CAD build for the part. Positions are in the model's coordinates, mm. A direction names the side the tool comes from. Give positions to 0.01 mm unless a question says otherwise; leave off trailing zeros. Loops run counter-clockwise (first coordinate to the right, second up) from the corner with the lowest first, then second, coordinate; pieces in that order, holes last. Notation, with made-up numbers: (62.25, 30) -> (108.25, 30) arc R29 cw to (108.25, 66) -> close; hole circle Ø4 at (87.25, 20.25). An arc over 180 degrees is marked (long way). Use one line per item in the form item = value.
```python
from build123d import *
from build123d import SkipClean  # not in build123d's __all__

# Parameters (mm, degrees)
F1_DEPTH = 6
F2_DEPTH = 8
F3_DEPTH = 15
F4_DEPTH = 72
F5_DEPTH = 96
F6_DEPTH = 40
F7_R     = 4
F8_DEPTH = 25


# Not quite as in the source:
# - after a boolean that leaves OpenCascade's solid faulty, fix() repairs it


with BuildPart() as f1:
    # F0 (on Front) → F1 (new body)
    with BuildSketch(Plane.XZ):
        with BuildLine():
            Line((-21, 7.2767180102), (-21, 19.3786125664))
            ThreePointArc((-21, 19.3786125664), (-22.4015502975, 17.7398187497), (-23.6755279772, 16))
            Line((-23.6755279772, 16), (-23.6755279772, -16))
            ThreePointArc((-23.6755279772, -16), (-22.4015502975, -17.7398187497), (-21, -19.3786125664))
            Line((-21, -19.3786125664), (-21, -7.2767180102))
            ThreePointArc((-21, -7.2767180102), (-22.225, 0), (-21, 7.2767180102))
        make_face()
        with BuildLine():
            Line((-21, -7.2767180102), (-21, 7.2767180102))
            ThreePointArc((-21, 7.2767180102), (-22.225, 0), (-21, -7.2767180102))
        make_face()
        with BuildLine():
            Line((21, 7.2767180102), (21, 19.3786125664))
            ThreePointArc((21, 19.3786125664), (0, 28.575), (-21, 19.3786125664))
            Line((-21, 19.3786125664), (-21, 7.2767180102))
            ThreePointArc((-21, 7.2767180102), (0, 22.225), (21, 7.2767180102))
        make_face()
        with BuildLine():
            Line((21, -7.2767180102), (21, 7.2767180102))
            ThreePointArc((21, 7.2767180102), (0, 22.225), (-21, 7.2767180102))
            Line((-21, 7.2767180102), (-21, -7.2767180102))
            ThreePointArc((-21, -7.2767180102), (0, -22.225), (21, -7.2767180102))
        make_face()
        with BuildLine():
            ThreePointArc((10.8581766425, 9.29), (13.4046157017, 4.9518055181), (14.29, 0))
            ThreePointArc((14.29, 0), (-4.9518055181, -13.4046157017), (-10.8581766425, 9.29))
            ThreePointArc((-10.8581766425, 9.29), (0, 14.29), (10.8581766425, 9.29))
        make_face(mode=Mode.SUBTRACT)
        with BuildLine():
            ThreePointArc((-21, -19.3786125664), (0, -28.575), (21, -19.3786125664))
            Line((21, -19.3786125664), (21, -7.2767180102))
            ThreePointArc((21, -7.2767180102), (0, -22.225), (-21, -7.2767180102))
            Line((-21, -7.2767180102), (-21, -19.3786125664))
        make_face()
        with BuildLine():
            ThreePointArc((22.225, 0), (21.9166104245, 3.6895545124), (21, 7.2767180102))
            Line((21, 7.2767180102), (21, -7.2767180102))
            ThreePointArc((21, -7.2767180102), (21.9166104245, -3.6895545124), (22.225, 0))
        make_face()
        with BuildLine():
            Line((23.6755279772, -16), (23.6755279772, 16))
            ThreePointArc((23.6755279772, 16), (22.4015502975, 17.7398187497), (21, 19.3786125664))
            Line((21, 19.3786125664), (21, 7.2767180102))
            ThreePointArc((21, 7.2767180102), (21.9166104245, 3.6895545124), (22.225, 0))
            ThreePointArc((22.225, 0), (21.9166104245, -3.6895545124), (21, -7.2767180102))
            Line((21, -7.2767180102), (21, -19.3786125664))
            ThreePointArc((21, -19.3786125664), (22.4015502975, -17.7398187497), (23.6755279772, -16))
        make_face()
        with BuildLine():
            ThreePointArc((-10.8581766425, 9.29), (-4.9518055181, -13.4046157017), (14.29, 0))
            ThreePointArc((14.29, 0), (13.4046157017, 4.9518055181), (10.8581766425, 9.29))
            Line((10.8581766425, 9.29), (-10.8581766425, 9.29))
        make_face()
        with BuildLine():
            Line((-10.8581766425, 9.29), (10.8581766425, 9.29))
            ThreePointArc((10.8581766425, 9.29), (0, 14.29), (-10.8581766425, 9.29))
        make_face()
    extrude(amount=-F1_DEPTH)

    # F0 (on Front) → F2 (join)
    with BuildSketch(Plane.XZ):
        with BuildLine():
            Line((21, -7.2767180102), (21, 7.2767180102))
            ThreePointArc((21, 7.2767180102), (0, 22.225), (-21, 7.2767180102))
            Line((-21, 7.2767180102), (-21, -7.2767180102))
            ThreePointArc((-21, -7.2767180102), (0, -22.225), (21, -7.2767180102))
        make_face()
        with BuildLine():
            ThreePointArc((10.8581766425, 9.29), (13.4046157017, 4.9518055181), (14.29, 0))
            ThreePointArc((14.29, 0), (-4.9518055181, -13.4046157017), (-10.8581766425, 9.29))
            ThreePointArc((-10.8581766425, 9.29), (0, 14.29), (10.8581766425, 9.29))
        make_face(mode=Mode.SUBTRACT)
        with BuildLine():
            ThreePointArc((-10.8581766425, 9.29), (-4.9518055181, -13.4046157017), (14.29, 0))
            ThreePointArc((14.29, 0), (13.4046157017, 4.9518055181), (10.8581766425, 9.29))
            Line((10.8581766425, 9.29), (-10.8581766425, 9.29))
        make_face()
        with BuildLine():
            Line((21, 7.2767180102), (21, 19.3786125664))
            ThreePointArc((21, 19.3786125664), (0, 28.575), (-21, 19.3786125664))
            Line((-21, 19.3786125664), (-21, 7.2767180102))
            ThreePointArc((-21, 7.2767180102), (0, 22.225), (21, 7.2767180102))
        make_face()
        with BuildLine():
            ThreePointArc((-21, -19.3786125664), (0, -28.575), (21, -19.3786125664))
            Line((21, -19.3786125664), (21, -7.2767180102))
            ThreePointArc((21, -7.2767180102), (0, -22.225), (-21, -7.2767180102))
            Line((-21, -7.2767180102), (-21, -19.3786125664))
        make_face()
        with BuildLine():
            ThreePointArc((23.6755279772, -16), (27.3226905424, -8.3666723687), (28.575, 0))
            ThreePointArc((28.575, 0), (27.3226905424, 8.3666723687), (23.6755279772, 16))
            Line((23.6755279772, 16), (23.6755279772, -16))
        make_face()
        with BuildLine():
            Line((-23.6755279772, -16), (-23.6755279772, 16))
            ThreePointArc((-23.6755279772, 16), (-28.575, 0), (-23.6755279772, -16))
        make_face()
        with BuildLine():
            Line((23.6755279772, -16), (23.6755279772, 16))
            ThreePointArc((23.6755279772, 16), (22.4015502975, 17.7398187497), (21, 19.3786125664))
            Line((21, 19.3786125664), (21, 7.2767180102))
            ThreePointArc((21, 7.2767180102), (21.9166104245, 3.6895545124), (22.225, 0))
            ThreePointArc((22.225, 0), (21.9166104245, -3.6895545124), (21, -7.2767180102))
            Line((21, -7.2767180102), (21, -19.3786125664))
            ThreePointArc((21, -19.3786125664), (22.4015502975, -17.7398187497), (23.6755279772, -16))
        make_face()
        with BuildLine():
            Line((-21, 7.2767180102), (-21, 19.3786125664))
            ThreePointArc((-21, 19.3786125664), (-22.4015502975, 17.7398187497), (-23.6755279772, 16))
            Line((-23.6755279772, 16), (-23.6755279772, -16))
            ThreePointArc((-23.6755279772, -16), (-22.4015502975, -17.7398187497), (-21, -19.3786125664))
            Line((-21, -19.3786125664), (-21, -7.2767180102))
            ThreePointArc((-21, -7.2767180102), (-22.225, 0), (-21, 7.2767180102))
        make_face()
        with BuildLine():
            Line((-10.8581766425, 9.29), (10.8581766425, 9.29))
            ThreePointArc((10.8581766425, 9.29), (0, 14.29), (-10.8581766425, 9.29))
        make_face()
        with BuildLine():
            Line((-21, -7.2767180102), (-21, 7.2767180102))
            ThreePointArc((-21, 7.2767180102), (-22.225, 0), (-21, -7.2767180102))
        make_face()
        with BuildLine():
            ThreePointArc((22.225, 0), (21.9166104245, 3.6895545124), (21, 7.2767180102))
            Line((21, 7.2767180102), (21, -7.2767180102))
            ThreePointArc((21, -7.2767180102), (21.9166104245, -3.6895545124), (22.225, 0))
        make_face()
    with SkipClean():  # cleaning this boolean's faces spoils the solid; the shape is the same uncleaned
        extrude(amount=F2_DEPTH)

    # F0 (on Front) → F3 (join)
    with BuildSketch(Plane.XZ):
        with BuildLine():
            Line((21, -7.2767180102), (21, 7.2767180102))
            ThreePointArc((21, 7.2767180102), (0, 22.225), (-21, 7.2767180102))
            Line((-21, 7.2767180102), (-21, -7.2767180102))
            ThreePointArc((-21, -7.2767180102), (0, -22.225), (21, -7.2767180102))
        make_face()
        with BuildLine():
            ThreePointArc((10.8581766425, 9.29), (13.4046157017, 4.9518055181), (14.29, 0))
            ThreePointArc((14.29, 0), (-4.9518055181, -13.4046157017), (-10.8581766425, 9.29))
            ThreePointArc((-10.8581766425, 9.29), (0, 14.29), (10.8581766425, 9.29))
        make_face(mode=Mode.SUBTRACT)
        with BuildLine():
            ThreePointArc((-10.8581766425, 9.29), (-4.9518055181, -13.4046157017), (14.29, 0))
            ThreePointArc((14.29, 0), (13.4046157017, 4.9518055181), (10.8581766425, 9.29))
            Line((10.8581766425, 9.29), (-10.8581766425, 9.29))
        make_face()
        with BuildLine():
            Line((21, 7.2767180102), (21, 19.3786125664))
            ThreePointArc((21, 19.3786125664), (0, 28.575), (-21, 19.3786125664))
            Line((-21, 19.3786125664), (-21, 7.2767180102))
            ThreePointArc((-21, 7.2767180102), (0, 22.225), (21, 7.2767180102))
        make_face()
        with BuildLine():
            ThreePointArc((-21, -19.3786125664), (0, -28.575), (21, -19.3786125664))
            Line((21, -19.3786125664), (21, -7.2767180102))
            ThreePointArc((21, -7.2767180102), (0, -22.225), (-21, -7.2767180102))
            Line((-21, -7.2767180102), (-21, -19.3786125664))
        make_face()
        with BuildLine():
            Line((-10.8581766425, 9.29), (10.8581766425, 9.29))
            ThreePointArc((10.8581766425, 9.29), (0, 14.29), (-10.8581766425, 9.29))
        make_face()
    extrude(amount=F3_DEPTH)

    add(f1.part.fix(), mode=Mode.REPLACE)

    # F0 (on Front) → F4 (join)
    with BuildSketch(Plane.XZ):
        with BuildLine():
            ThreePointArc((-10.8581766425, 9.29), (-4.9518055181, -13.4046157017), (14.29, 0))
            ThreePointArc((14.29, 0), (13.4046157017, 4.9518055181), (10.8581766425, 9.29))
            Line((10.8581766425, 9.29), (-10.8581766425, 9.29))
        make_face()
        with BuildLine():
            Line((-10.8581766425, 9.29), (10.8581766425, 9.29))
            ThreePointArc((10.8581766425, 9.29), (0, 14.29), (-10.8581766425, 9.29))
        make_face()
    extrude(amount=F4_DEPTH)

    # F0 (on Front) → F5 (join)
    with BuildSketch(Plane.XZ):
        with BuildLine():
            ThreePointArc((-10.8581766425, 9.29), (-4.9518055181, -13.4046157017), (14.29, 0))
            ThreePointArc((14.29, 0), (13.4046157017, 4.9518055181), (10.8581766425, 9.29))
            Line((10.8581766425, 9.29), (-10.8581766425, 9.29))
        make_face()
    extrude(amount=F5_DEPTH)

    # F0 (on Front) → F6 (join)
    with BuildSketch(Plane.XZ):
        with BuildLine():
            Line((21, -7.2767180102), (21, 7.2767180102))
            ThreePointArc((21, 7.2767180102), (0, 22.225), (-21, 7.2767180102))
            Line((-21, 7.2767180102), (-21, -7.2767180102))
            ThreePointArc((-21, -7.2767180102), (0, -22.225), (21, -7.2767180102))
        make_face()
        with BuildLine():
            ThreePointArc((10.8581766425, 9.29), (13.4046157017, 4.9518055181), (14.29, 0))
            ThreePointArc((14.29, 0), (-4.9518055181, -13.4046157017), (-10.8581766425, 9.29))
            ThreePointArc((-10.8581766425, 9.29), (0, 14.29), (10.8581766425, 9.29))
        make_face(mode=Mode.SUBTRACT)
        with BuildLine():
            ThreePointArc((-10.8581766425, 9.29), (-4.9518055181, -13.4046157017), (14.29, 0))
            ThreePointArc((14.29, 0), (13.4046157017, 4.9518055181), (10.8581766425, 9.29))
            Line((10.8581766425, 9.29), (-10.8581766425, 9.29))
        make_face()
        with BuildLine():
            Line((-10.8581766425, 9.29), (10.8581766425, 9.29))
            ThreePointArc((10.8581766425, 9.29), (0, 14.29), (-10.8581766425, 9.29))
        make_face()
    extrude(amount=F6_DEPTH)

    # F7 (on face) → F8 (cut)
    with BuildSketch(Plane.XY.offset(9.29)):
        with Locations((0, -84)):
            Circle(F7_R)
    extrude(amount=-F8_DEPTH, mode=Mode.SUBTRACT)


solid = f1.part
```
1. Cut at B-B, the plane z = 6. Write the cut outline in (x, y), then the cut area to 3 significant figures.
Result sheet:
outline = (-27.94, -8) -> (-21, -8) -> (-21, -40) -> (-12.97, -40) -> (-12.97, -96) -> (12.97, -96) -> (12.97, -40) -> (21, -40) -> (21, -8) -> (27.94, -8) -> (27.94, 0) -> (23.68, 0) -> (23.68, 6) -> (-23.68, 6) -> (-23.68, 0) -> (-27.94, 0) -> close; hole circle Ø8 at (0, -84)
area = 3,480 mm^2
2. Mould opens along Y. For faces 6 (the cylindrical face through (0.38, -27.32, 22.22)), 7 (the cylindrical face through (-0.867, -87.905, -2.335)), 8 (the flat face through (0, 6, 0)), 9 (the flat face through (0, -40, -15)) say: pulls with the +Y half, pulls with the -Y half, needs draft (parallel to the pull), parting line crosses it, or undercut.
Result sheet:
face_6 = needs draft
face_7 = undercut
face_8 = pulls with the +Y half
face_9 = pulls with the -Y half
3. Cut at A-A, the plane x = 0. Write the cut outline in (y, z) (3 decimals), then the cut area to 3 significant figures.
Result sheet:
outline = (-96, -14.29) -> (-88, -14.29) -> (-88, 9.29) -> (-96, 9.29) -> close; (-80, -14.29) -> (-40, -14.29) -> (-40, -22.225) -> (-15, -22.225) -> (-15, -28.575) -> (6, -28.575) -> (6, 28.575) -> (-15, 28.575) -> (-15, 22.225) -> (-40, 22.225) -> (-40, 14.29) -> (-72, 14.29) -> (-72, 9.29) -> (-80, 9.29) -> close
area = 3,600 mm^2
4. Cut at C-C, the plane y = -84. Write the cut outline in (x, z), then the cut area to 3 significant figures.
Result sheet:
outline = (-10.86, 9.29) arc R14.29 ccw to (-4, -13.72) -> (-4, 9.29) -> close; (4, -13.72) arc R14.29 ccw to (10.86, 9.29) -> (4, 9.29) -> close
area = 379 mm^2
5. Cut at D-D, the plane y = -47. Write the cut outline in (x, z), then the cut area to 3 significant figures.
Result sheet:
outline = circle Ø28.58 at (0, 0)
area = 642 mm^2
6. Tool access for faces 1 (the flat face through (26, 0, 0)), 2 (the flat face through (-26, 0, 0)), 3 (the flat face through (-24, -8, 0)), 4 (the flat face through (0, -72, 11)), 5 (the flat face through (24, -8, 0)): list every direction of +Z, -Z, +X, -X, +Y, -Y with a clear straight run to the whole face (end or side of a thin tool).
Result sheet:
face_1 = +Z, -Z, +X, +Y
face_2 = +Z, -Z, -X, +Y
face_3 = +Z, -Z, -X, -Y
face_4 = +Z, +X, -X, -Y
face_5 = +Z, -Z, +X, -Y
7. Drill centre lines: line 1 (Y direction, x = 0, z = -9); line 2 (X direction, y = -36, z = -1); line 3 (Y direction, x = 26, z = -10.5). Where is each one in solid material? Low to high.
Result sheet:
line_1 = -96 to -88, -80 to 6
line_2 = -21 to 21
line_3 = -8 to 0
8. Drop flat-ended pins along their axis: P1, Ø3, axis at y = -44, z = 5.5, coming from the +X side; P2, Ø5.5, axis at x = 26.5, z = 3.5, coming from the +Y side; P3, Ø17, axis at x = -10, z = -22.5, coming from the -Y side. Give the stop position or say it passes through.
Result sheet:
P1 = 13.72
P2 = 0
P3 = -40
